```python
from build123d import *

# Parameters (mm, degrees)
BOSS_EXTRUDE1_DEPTH = 130


with BuildPart() as part:
    # Sketch1 → Boss-Extrude1 (new body, symmetric)
    with BuildSketch(Plane(origin=(0, 0, 0), x_dir=(1, 0, 0), z_dir=(0, 1, 0))):
        with BuildLine():
            Line((-27.932619, -6.859853), (-27.932619, 5.140147))
            ThreePointArc((-27.932619, 5.140147), (-26.761046, 7.968574), (-23.932619, 9.140147))
            Line((-23.932619, 9.140147), (-11.932619, 9.140147))
            Line((-11.932619, 9.140147), (-11.932619, 4.640147))
            Line((-11.932619, 4.640147), (-19.182619, 4.640147))
            Line((-19.182619, 4.640147), (-19.182619, 3.140147))
            Line((-19.182619, 3.140147), (-12.932619, -3.109853))
            Line((-12.932619, -3.109853), (-7.932619, -3.109853))
            Line((-7.932619, -3.109853), (-2.932619, -3.109853))
            Line((-2.932619, -3.109853), (3.317381, 3.140147))
            Line((3.317381, 3.140147), (3.317381, 4.640147))
            Line((3.317381, 4.640147), (-3.932619, 4.640147))
            Line((-3.932619, 4.640147), (-3.932619, 9.140147))
            Line((-3.932619, 9.140147), (8.067381, 9.140147))
            ThreePointArc((8.067381, 9.140147), (10.895808, 7.968574), (12.067381, 5.140147))
            Line((12.067381, 5.140147), (12.067381, -6.859853))
            Line((12.067381, -6.859853), (7.567381, -6.859853))
            Line((7.567381, -6.859853), (7.567381, 0.390147))
            Line((7.567381, 0.390147), (6.067381, 0.390147))
            Line((6.067381, 0.390147), (-0.182619, -5.859853))
            Line((-0.182619, -5.859853), (-0.182619, -10.859853))
            Line((-0.182619, -10.859853), (-0.182619, -15.859853))
            Line((-0.182619, -15.859853), (6.067381, -22.109853))
            Line((6.067381, -22.109853), (7.567381, -22.109853))
            Line((7.567381, -22.109853), (7.567381, -14.859853))
            Line((7.567381, -14.859853), (12.067381, -14.859853))
            Line((12.067381, -14.859853), (12.067381, -26.859853))
            ThreePointArc((12.067381, -26.859853), (10.895808, -29.68828), (8.067381, -30.859853))
            Line((8.067381, -30.859853), (-3.932619, -30.859853))
            Line((-3.932619, -30.859853), (-3.932619, -26.359853))
            Line((-3.932619, -26.359853), (3.317381, -26.359853))
            Line((3.317381, -26.359853), (3.317381, -24.859853))
            Line((3.317381, -24.859853), (-2.932619, -18.609853))
            Line((-2.932619, -18.609853), (-7.932619, -18.609853))
            Line((-7.932619, -18.609853), (-12.932619, -18.609853))
            Line((-12.932619, -18.609853), (-19.182619, -24.859853))
            Line((-19.182619, -24.859853), (-19.182619, -26.359853))
            Line((-19.182619, -26.359853), (-11.932619, -26.359853))
            Line((-11.932619, -26.359853), (-11.932619, -30.859853))
            Line((-11.932619, -30.859853), (-23.932619, -30.859853))
            ThreePointArc((-23.932619, -30.859853), (-26.761046, -29.68828), (-27.932619, -26.859853))
            Line((-27.932619, -26.859853), (-27.932619, -14.859853))
            Line((-27.932619, -14.859853), (-23.432619, -14.859853))
            Line((-23.432619, -14.859853), (-23.432619, -22.109853))
            Line((-23.432619, -22.109853), (-21.932619, -22.109853))
            Line((-21.932619, -22.109853), (-15.682619, -15.859853))
            Line((-15.682619, -15.859853), (-15.682619, -10.859853))
            Line((-15.682619, -10.859853), (-15.682619, -5.859853))
            Line((-15.682619, -5.859853), (-21.932619, 0.390147))
            Line((-21.932619, 0.390147), (-23.432619, 0.390147))
            Line((-23.432619, 0.390147), (-23.432619, -6.859853))
            Line((-23.432619, -6.859853), (-27.932619, -6.859853))
        make_face()
        with BuildLine():
            Line((-25.932619, 2.390147), (-25.932619, 5.140147))
            ThreePointArc((-25.932619, 5.140147), (-25.346832, 6.554361), (-23.932619, 7.140147))
            Line((-23.932619, 7.140147), (-21.182619, 7.140147))
            Line((-21.182619, 7.140147), (-21.182619, 3.097254))
            Line((-21.182619, 3.097254), (-20.734396, 2.649031))
            Line((-20.734396, 2.649031), (-21.441502, 1.941924))
            Line((-21.441502, 1.941924), (-21.889726, 2.390147))
            Line((-21.889726, 2.390147), (-25.932619, 2.390147))
        make_face(mode=Mode.SUBTRACT)
        with BuildLine():
            Line((-20.380842, 0.881264), (-13.682619, -5.816959))
            Line((-13.682619, -5.816959), (-13.682619, -7.955115))
            Line((-13.682619, -7.955115), (-13.182619, -7.955115))
            Line((-13.182619, -7.955115), (-12.002324, -7.955115))
            ThreePointArc((-12.002324, -7.955115), (-11.468153, -7.324319), (-10.837356, -6.790148))
            Line((-10.837356, -6.790148), (-10.837356, -5.609853))
            Line((-10.837356, -5.609853), (-10.837356, -5.109853))
            Line((-10.837356, -5.109853), (-12.975512, -5.109853))
            Line((-12.975512, -5.109853), (-19.673735, 1.588371))
            Line((-19.673735, 1.588371), (-20.380842, 0.881264))
        make_face(mode=Mode.SUBTRACT)
        with BuildLine():
            Line((10.067381, 2.390147), (10.067381, 5.140147))
            ThreePointArc((10.067381, 5.140147), (9.481595, 6.554361), (8.067381, 7.140147))
            Line((8.067381, 7.140147), (5.317381, 7.140147))
            Line((5.317381, 7.140147), (5.317381, 3.097254))
            Line((5.317381, 3.097254), (4.869158, 2.649031))
            Line((4.869158, 2.649031), (5.576265, 1.941924))
            Line((5.576265, 1.941924), (6.024488, 2.390147))
            Line((6.024488, 2.390147), (10.067381, 2.390147))
        make_face(mode=Mode.SUBTRACT)
        with BuildLine():
            Line((-2.182619, -5.816959), (-2.182619, -7.955115))
            Line((-2.182619, -7.955115), (-2.682619, -7.955115))
            Line((-2.682619, -7.955115), (-3.862914, -7.955115))
            ThreePointArc((-3.862914, -7.955115), (-4.397085, -7.324319), (-5.027881, -6.790148))
            Line((-5.027881, -6.790148), (-5.027881, -5.609853))
            Line((-5.027881, -5.609853), (-5.027881, -5.109853))
            Line((-5.027881, -5.109853), (-2.889726, -5.109853))
            Line((-2.889726, -5.109853), (3.808498, 1.588371))
            Line((3.808498, 1.588371), (4.515604, 0.881264))
            Line((4.515604, 0.881264), (-2.182619, -5.816959))
        make_face(mode=Mode.SUBTRACT)
        with BuildLine():
            Line((5.317381, -28.859853), (8.067381, -28.859853))
            ThreePointArc((8.067381, -28.859853), (9.481595, -28.274066), (10.067381, -26.859853))
            Line((10.067381, -26.859853), (10.067381, -24.109853))
            Line((10.067381, -24.109853), (6.024488, -24.109853))
            Line((6.024488, -24.109853), (5.576265, -23.661629))
            Line((5.576265, -23.661629), (4.869158, -24.368736))
            Line((4.869158, -24.368736), (5.317381, -24.816959))
            Line((5.317381, -24.816959), (5.317381, -28.859853))
        make_face(mode=Mode.SUBTRACT)
        with BuildLine():
            Line((-2.889726, -16.609853), (-5.027881, -16.609853))
            Line((-5.027881, -16.609853), (-5.027881, -16.109853))
            Line((-5.027881, -16.109853), (-5.027881, -14.929558))
            ThreePointArc((-5.027881, -14.929558), (-4.397085, -14.395387), (-3.862914, -13.76459))
            Line((-3.862914, -13.76459), (-2.682619, -13.76459))
            Line((-2.682619, -13.76459), (-2.182619, -13.76459))
            Line((-2.182619, -13.76459), (-2.182619, -15.902746))
            Line((-2.182619, -15.902746), (4.515604, -22.600969))
            Line((4.515604, -22.600969), (3.808498, -23.308076))
            Line((3.808498, -23.308076), (-2.889726, -16.609853))
        make_face(mode=Mode.SUBTRACT)
        with BuildLine():
            Line((-25.932619, -24.109853), (-25.932619, -26.859853))
            ThreePointArc((-25.932619, -26.859853), (-25.346832, -28.274066), (-23.932619, -28.859853))
            Line((-23.932619, -28.859853), (-21.182619, -28.859853))
            Line((-21.182619, -28.859853), (-21.182619, -24.816959))
            Line((-21.182619, -24.816959), (-20.734396, -24.368736))
            Line((-20.734396, -24.368736), (-21.441502, -23.661629))
            Line((-21.441502, -23.661629), (-21.889726, -24.109853))
            Line((-21.889726, -24.109853), (-25.932619, -24.109853))
        make_face(mode=Mode.SUBTRACT)
        with BuildLine():
            Line((-13.682619, -15.902746), (-13.682619, -13.76459))
            Line((-13.682619, -13.76459), (-13.182619, -13.76459))
            Line((-13.182619, -13.76459), (-12.002324, -13.76459))
            ThreePointArc((-12.002324, -13.76459), (-11.468153, -14.395387), (-10.837356, -14.929558))
            Line((-10.837356, -14.929558), (-10.837356, -16.109853))
            Line((-10.837356, -16.109853), (-10.837356, -16.609853))
            Line((-10.837356, -16.609853), (-12.975512, -16.609853))
            Line((-12.975512, -16.609853), (-19.673735, -23.308076))
            Line((-19.673735, -23.308076), (-20.380842, -22.600969))
            Line((-20.380842, -22.600969), (-13.682619, -15.902746))
        make_face(mode=Mode.SUBTRACT)
        with BuildLine():
            ThreePointArc((-11.332619, -10.859853), (-10.336782, -8.45569), (-7.932619, -7.459853))
            ThreePointArc((-7.932619, -7.459853), (-5.528456, -8.45569), (-4.532619, -10.859853))
            ThreePointArc((-4.532619, -10.859853), (-5.528456, -13.264016), (-7.932619, -14.259853))
            ThreePointArc((-7.932619, -14.259853), (-10.336782, -13.264016), (-11.332619, -10.859853))
        make_face(mode=Mode.SUBTRACT)
    extrude(amount=BOSS_EXTRUDE1_DEPTH, both=True)


solid = part.part
```
Input: part model. Units: mm. Frame: model coordinates. A direction names the side the tool comes from. Coordinates: 2 decimals unless noted, no trailing zeros. One line per item, written item: value.
(1) Reachability of faces 1 (the flat face through (-3.933, 2, 29)), 2 (the cylindrical face through (-26.73, 1.82, 29.72)), 3 (the flat face through (-16, 2, -4.64)), 4 (the flat face through (-26, 2, 14.86)) from +Z, -Z, +X, -X, +Y, -Y: full face, straight path, thin tool, end or side. Return the list, or none.
Filled in:
face 1: +Z, +Y, -Y
face 2: +Z, -X, +Y, -Y
face 3: +Y, -Y
face 4: -X, +Y, -Y
(2) Pull-direction query (Z, two-part tool) for faces 5 (the flat face through (10, 2, 14.86)), 6 (the flat face through (-18, 2, 30.86)), 7 (the flat face through (12.067, 2, 1)); classes: +Z half, -Z half, draft (parallel to the pull), parting line (faces both ways), or undercut.
Filled in:
face 5: undercut
face 6: +Z half
face 7: draft
(3) Section A-A (y = 104.5). Give the number of separate pieces and of enclosed holes in the cut face, and give its area (3 significant figures).
Filled in:
separate pieces: 1
enclosed holes: 9
area: 710 mm^2
(4) Line query: line 1 along Z through (x, y) = (-23, -115); line 2 along X through (y, z) = (-78, 6.5); line 3 along X through (y, z) = (-22, -4). Output: solid intervals per line, ascending. Write a range as from..to.
Filled in:
line 1: -9.14..-7.14, -2.39..-0.39, 22.11..24.11, 28.86..30.86
line 2: -27.93..-23.43, -15.68..-13.68, -10.84..-5.03, -2.18..-0.18, 7.57..12.07
line 3: -27.93..-25.93, -21.18..-19.18, 3.32..5.32, 10.07..12.07
